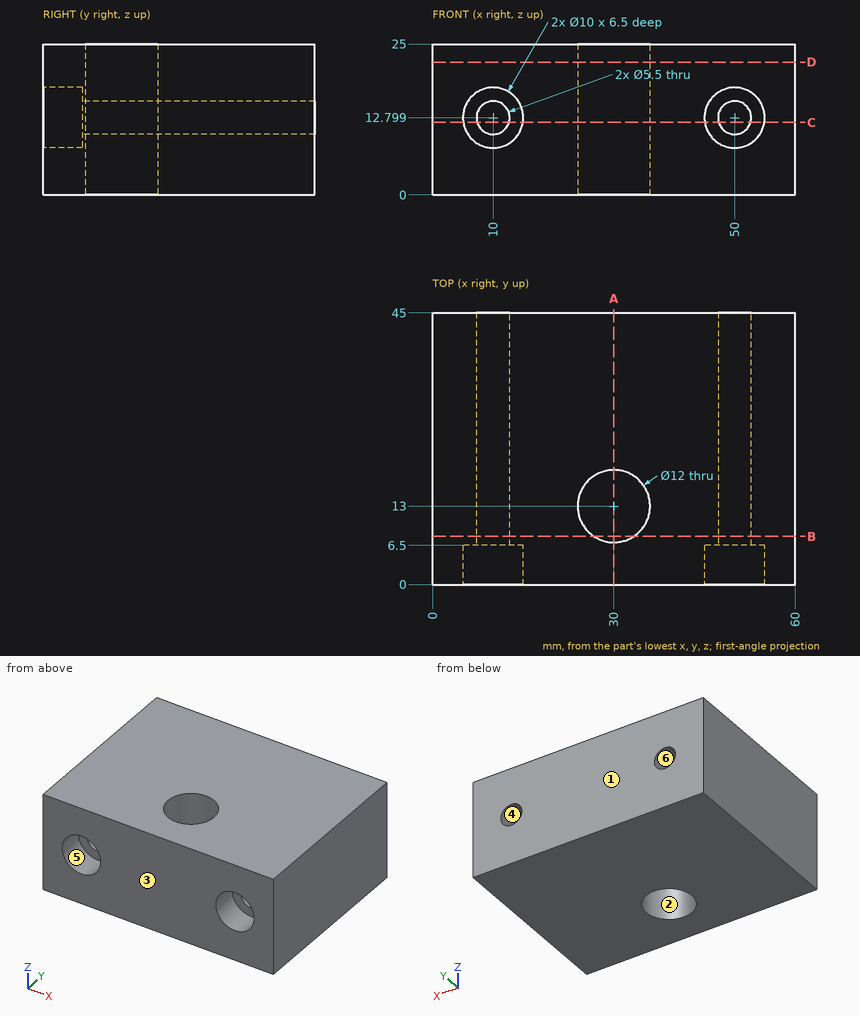
The drawing under review shows one solid part. Ordinate dimensions are in mm from its lowest x, y, z. A direction names the side the tool comes from. Round coordinates to 2 decimals unless told otherwise and drop trailing zeros. Write each loop counter-clockwise with the first axis right and the second up, starting at its lowest first coordinate (ties: lowest second). Pieces come first, ordered by that corner, then holes. Notation, with made-up numbers: (42.5, 38) - (85.5, 38) arc R20 ccw to (85.5, 74) - close; hole circle Ø4 at (36, 8.25). An arc over 180 degrees is marked (long way). Use a Markdown table: item, result. Add a question column.
1. We need section C-C (z = 12). State the section outline as (x, y) points.
2. Clearance check with flat-ended pins moving along their axes: pin 1 (6 mm diameter, centred on x = 50, z = 12.8, fed in from +Y); pin 2 (3 mm diameter, centred on x = 50, z = 11, fed in from -Y); pin 3 (5 mm diameter, centred on x = 50, z = 12.8, fed in from -Y). State where each tip first meets the part, or that it passes through.
3. We need section D-D (z = 22). State the section outline as (x, y) points.
4. We need section A-A (x = 30). State the section outline as (y, z) points.
5. We need section B-B (y = 8). State the section outline as (x, z) points.
6. For the marked faces 5 and 6, list the 3-axis set-ups (+Z, -Z, +X, -X, +Y, -Y) from which the entire face can be reached by the end or side of a thin tool; tool diameter is ignored.
7. Wall thickness on probe 1 along X at (y, z) = (28.5, 12.25); probe 2 along X at (y, z) = (6, 10.5); probe 3 along Y at (x, z) = (30, 18.5): over which ranges is each line inside the solid? List them lowest first.
8. Mouldability with a two-part tool opening along Y and no side actions: class the marked faces 1, 2, 3 and 4 as +Y half, -Y half, draft (parallel to the pull), parting line (faces both ways), or undercut.
Output:
| question | item | result |
|---|---|---|
| 1 | outline | (0, 0) - (5.06, 0) - (5.06, 6.5) - (7.37, 6.5) - (7.37, 45) - (0, 45) - close; (12.63, 6.5) - (14.94, 6.5) - (14.94, 0) - (45.06, 0) - (45.06, 6.5) - (47.37, 6.5) - (47.37, 45) - (12.63, 45) - close; (52.63, 6.5) - (54.94, 6.5) - (54.94, 0) - (60, 0) - (60, 45) - (52.63, 45) - close; hole circle Ø12 at (30, 13) |
| 2 | pin 1 | stops at y = 45 |
| 2 | pin 2 | stops at y = 6.5 |
| 2 | pin 3 | passes through |
| 3 | outline | (0, 0) - (60, 0) - (60, 45) - (0, 45) - close; hole circle Ø12 at (30, 13) |
| 4 | outline | (0, 0) - (7, 0) - (7, 25) - (0, 25) - close; (19, 0) - (45, 0) - (45, 25) - (19, 25) - close |
| 5 | outline | (0, 0) - (26.68, 0) - (26.68, 25) - (0, 25) - close; (33.32, 0) - (60, 0) - (60, 25) - (33.32, 25) - close; hole circle Ø5.5 at (10, 12.8); hole circle Ø5.5 at (50, 12.8) |
| 6 | face 5 | -Y |
| 6 | face 6 | +Y, -Y |
| 7 | probe 1 | x = 0 to 7.31, 12.69 to 47.31, 52.69 to 60 |
| 7 | probe 2 | x = 0 to 5.56, 14.44 to 45.56, 54.44 to 60 |
| 7 | probe 3 | y = 0 to 7, 19 to 45 |
| 8 | face 1 | +Y half |
| 8 | face 2 | undercut |
| 8 | face 3 | -Y half |
| 8 | face 4 | draft |
